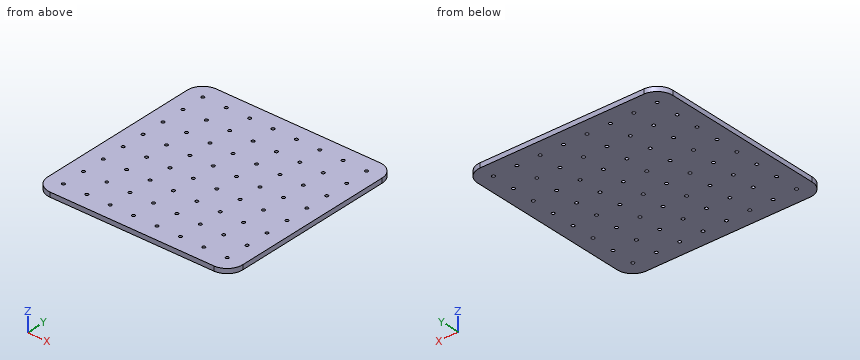
```python
from build123d import *

# Parameters (mm, degrees)
F0_R     = 2
F1_DEPTH = 6


with BuildPart() as f1:
    # F0 (on Top) → F1 (new body)
    with BuildSketch(Plane.XY):
        with BuildLine():
            Line((105, 125), (-105, 125))
            ThreePointArc((-105, 125), (-119.142136, 119.142136), (-125, 105))
            Line((-125, 105), (-125, -105))
            ThreePointArc((-125, -105), (-119.142136, -119.142136), (-105, -125))
            Line((-105, -125), (105, -125))
            ThreePointArc((105, -125), (119.142136, -119.142136), (125, -105))
            Line((125, -105), (125, 105))
            ThreePointArc((125, 105), (119.142136, 119.142136), (105, 125))
        make_face()
        with Locations((-105, -105)):
            Circle(F0_R, mode=Mode.SUBTRACT)
        with Locations((-75, -105)):
            Circle(F0_R, mode=Mode.SUBTRACT)
        with Locations((-105, -75)):
            Circle(F0_R, mode=Mode.SUBTRACT)
        with Locations((-75, -75)):
            Circle(F0_R, mode=Mode.SUBTRACT)
        with Locations((-45, -105)):
            Circle(F0_R, mode=Mode.SUBTRACT)
        with Locations((-15, -105)):
            Circle(F0_R, mode=Mode.SUBTRACT)
        with Locations((-45, -75)):
            Circle(F0_R, mode=Mode.SUBTRACT)
        with Locations((-15, -75)):
            Circle(F0_R, mode=Mode.SUBTRACT)
        with Locations((-105, -45)):
            Circle(F0_R, mode=Mode.SUBTRACT)
        with Locations((-75, -45)):
            Circle(F0_R, mode=Mode.SUBTRACT)
        with Locations((-105, -15)):
            Circle(F0_R, mode=Mode.SUBTRACT)
        with Locations((-75, -15)):
            Circle(F0_R, mode=Mode.SUBTRACT)
        with Locations((-45, -45)):
            Circle(F0_R, mode=Mode.SUBTRACT)
        with Locations((-15, -45)):
            Circle(F0_R, mode=Mode.SUBTRACT)
        with Locations((-45, -15)):
            Circle(F0_R, mode=Mode.SUBTRACT)
        with Locations((-15, -15)):
            Circle(F0_R, mode=Mode.SUBTRACT)
        with Locations((15, -105)):
            Circle(F0_R, mode=Mode.SUBTRACT)
        with Locations((45, -105)):
            Circle(F0_R, mode=Mode.SUBTRACT)
        with Locations((15, -75)):
            Circle(F0_R, mode=Mode.SUBTRACT)
        with Locations((45, -75)):
            Circle(F0_R, mode=Mode.SUBTRACT)
        with Locations((75, -105)):
            Circle(F0_R, mode=Mode.SUBTRACT)
        with Locations((105, -105)):
            Circle(F0_R, mode=Mode.SUBTRACT)
        with Locations((75, -75)):
            Circle(F0_R, mode=Mode.SUBTRACT)
        with Locations((105, -75)):
            Circle(F0_R, mode=Mode.SUBTRACT)
        with Locations((15, -45)):
            Circle(F0_R, mode=Mode.SUBTRACT)
        with Locations((45, -45)):
            Circle(F0_R, mode=Mode.SUBTRACT)
        with Locations((15, -15)):
            Circle(F0_R, mode=Mode.SUBTRACT)
        with Locations((45, -15)):
            Circle(F0_R, mode=Mode.SUBTRACT)
        with Locations((75, -45)):
            Circle(F0_R, mode=Mode.SUBTRACT)
        with Locations((105, -45)):
            Circle(F0_R, mode=Mode.SUBTRACT)
        with Locations((75, -15)):
            Circle(F0_R, mode=Mode.SUBTRACT)
        with Locations((105, -15)):
            Circle(F0_R, mode=Mode.SUBTRACT)
        with Locations((-105, 15)):
            Circle(F0_R, mode=Mode.SUBTRACT)
        with Locations((-75, 15)):
            Circle(F0_R, mode=Mode.SUBTRACT)
        with Locations((-105, 45)):
            Circle(F0_R, mode=Mode.SUBTRACT)
        with Locations((-75, 45)):
            Circle(F0_R, mode=Mode.SUBTRACT)
        with Locations((-45, 15)):
            Circle(F0_R, mode=Mode.SUBTRACT)
        with Locations((-15, 15)):
            Circle(F0_R, mode=Mode.SUBTRACT)
        with Locations((-45, 45)):
            Circle(F0_R, mode=Mode.SUBTRACT)
        with Locations((-15, 45)):
            Circle(F0_R, mode=Mode.SUBTRACT)
        with Locations((-105, 75)):
            Circle(F0_R, mode=Mode.SUBTRACT)
        with Locations((-75, 75)):
            Circle(F0_R, mode=Mode.SUBTRACT)
        with Locations((-105, 105)):
            Circle(F0_R, mode=Mode.SUBTRACT)
        with Locations((-75, 105)):
            Circle(F0_R, mode=Mode.SUBTRACT)
        with Locations((-45, 75)):
            Circle(F0_R, mode=Mode.SUBTRACT)
        with Locations((-15, 75)):
            Circle(F0_R, mode=Mode.SUBTRACT)
        with Locations((-45, 105)):
            Circle(F0_R, mode=Mode.SUBTRACT)
        with Locations((-15, 105)):
            Circle(F0_R, mode=Mode.SUBTRACT)
        with Locations((15, 15)):
            Circle(F0_R, mode=Mode.SUBTRACT)
        with Locations((45, 15)):
            Circle(F0_R, mode=Mode.SUBTRACT)
        with Locations((15, 45)):
            Circle(F0_R, mode=Mode.SUBTRACT)
        with Locations((45, 45)):
            Circle(F0_R, mode=Mode.SUBTRACT)
        with Locations((75, 15)):
            Circle(F0_R, mode=Mode.SUBTRACT)
        with Locations((105, 15)):
            Circle(F0_R, mode=Mode.SUBTRACT)
        with Locations((75, 45)):
            Circle(F0_R, mode=Mode.SUBTRACT)
        with Locations((105, 45)):
            Circle(F0_R, mode=Mode.SUBTRACT)
        with Locations((15, 75)):
            Circle(F0_R, mode=Mode.SUBTRACT)
        with Locations((45, 75)):
            Circle(F0_R, mode=Mode.SUBTRACT)
        with Locations((15, 105)):
            Circle(F0_R, mode=Mode.SUBTRACT)
        with Locations((45, 105)):
            Circle(F0_R, mode=Mode.SUBTRACT)
        with Locations((75, 75)):
            Circle(F0_R, mode=Mode.SUBTRACT)
        with Locations((105, 75)):
            Circle(F0_R, mode=Mode.SUBTRACT)
        with Locations((75, 105)):
            Circle(F0_R, mode=Mode.SUBTRACT)
        with Locations((105, 105)):
            Circle(F0_R, mode=Mode.SUBTRACT)
    extrude(amount=F1_DEPTH)


solid = f1.part
```
CAD build for the part. Positions are in the model's coordinates, mm. Round coordinates to 2 decimals unless told otherwise and drop trailing zeros. Answer in a Markdown table with one row per item. Add a question column.
(1) Probe L1, parallel to X at y = -110.5, z = 0.45. List the from-to ranges inside material, lowest first. Write a range as [from, to].
(2) Band-saw the part on A-A on z = 4.7. Count the separate pieces of the cut face and the enclosed holes in it, and give its area (3 significant figures).
(3) Drop a flat-ended pin along its axis: pin 1 Ø3.5 at (x, y) = (75, -105) entering from -Z. Give the stop position or say it passes through.
Data:
| question | item | result |
|---|---|---|
| 1 | L1 | x = [-124.23, 124.23] |
| 2 | separate pieces | 1 |
| 2 | enclosed holes | 64 |
| 2 | area | 61,400 mm^2 |
| 3 | pin 1 | passes through |
